Work out the finished part from the listing and answer in its coordinate system (mm). A direction names the side the tool comes from. Give positions to 0.01 mm unless a question says otherwise; leave off trailing zeros. Order: outer loops, then holes, each group sorted by start corner. A loop starts at its lowest first (then second) coordinate and runs counter-clockwise, first axis right, second up. Notation, with made-up numbers: (78, 82) - (121, 82) arc R19 cw to (121, 107) - close; hole circle Ø4 at (34.5, -30.5). An arc over 180 degrees is marked (long way). Put each result on its own line as item: value.
```python
from build123d import *

# Parameters (mm, degrees)
F1_DEPTH = 225
F3_D     = 16
F4_D     = 7


with BuildPart() as f1:
    # F0 (on Top) → F1 (new body, symmetric)
    with BuildSketch(Plane.XY):
        Polygon((-15, -15), (15, -15), (15, -14.1), (-14.1, -14.1), (-14.1, 15), (-15, 15), align=None)
    extrude(amount=F1_DEPTH, both=True)

    # F3 (through all)
    with Locations(Plane.XZ.offset(15)):
        with Locations((0, 175), (0, 85), (0, -5), (0, -95), (0, -185)):
            Hole(F3_D / 2)

    # F4 (through all)
    with Locations(Plane.XZ.offset(15)):
        with Locations((0, -155), (0, -65), (0, 25), (0, 115), (0, 205)):
            Hole(F4_D / 2)


solid = f1.part
```
(1) A tool of negligible diameter and unlimited length cuts with its end or side. For faces 1 (the face through (1.73, -14.54, -12.81)), 2 (the face through (0.7, -14.1, 3.2)), from which of +Z, -Z, +X, -X, +Y, -Y can it reach the whole face along a straight path? Write none if from no direction.
Geometry check:
face 1: +Y, -Y
face 2: +Z, -Z, +X, +Y
(2) Straight lines are drawn through the part: line 1 (Y direction, x = 12.5, z = 169); line 2 (X direction, y = -14.6, z = -155). For each, find the intervals that lie inside material, in ascending order.
Geometry check:
line 1: y = -15 to -14.1
line 2: x = -15 to -3.5, 3.5 to 15
(3) Given pin 1 (9.5 mm diameter, centred on x = 0, z = -95, fed in from +Y); pin 2 (3 mm diameter, centred on x = 5.5, z = -126.5, fed in from +Y); pin 3 (6 mm diameter, centred on y = 9, z = -179.5, fed in from +X), each flat-ended and moving along its own axis, determine where each tip first touches the part or whether it passes through.
Geometry check:
pin 1: passes through
pin 2: stops at y = -14.1
pin 3: stops at x = -14.1
(4) Section B-B, the plane z = 139 is taken. Write down the section's boundary in (x, y).
Geometry check:
outline: (-15, -15) - (15, -15) - (15, -14.1) - (-14.1, -14.1) - (-14.1, 15) - (-15, 15) - close
(5) Section C-C, the plane y = 4.75 is taken. Write down the section's boundary in (x, z), then the cut area to 3 significant figures.
Geometry check:
outline: (-15, -225) - (-14.1, -225) - (-14.1, 225) - (-15, 225) - close
area: 405 mm²
(6) Determine the mould class of faces 3 (the face through (-15, 0, 3)), 4 (the face through (1.041, -14.544, -87.068)), 5 (the face through (-14.5, -6.6, -225)) for opening direction X: pulls with the +X half, pulls with the -X half, needs draft (parallel to the pull), parting line crosses it, or undercut.
Geometry check:
face 3: pulls with the -X half
face 4: undercut
face 5: needs draft
(7) Section A-A, the plane z = -95 is taken. Write down the section's boundary in (x, y).
Geometry check:
outline: (-15, -15) - (-8, -15) - (-8, -14.1) - (-14.1, -14.1) - (-14.1, 15) - (-15, 15) - close; (8, -15) - (15, -15) - (15, -14.1) - (8, -14.1) - close
